The model under review builds one solid part; all positions refer to its coordinate system, in mm. A direction names the side the tool comes from. Round coordinates to 2 decimals unless told otherwise and drop trailing zeros. Loops run counter-clockwise (first coordinate to the right, second up) from the corner with the lowest first, then second, coordinate; pieces in that order, holes last. Notation, with made-up numbers: (-18.75, 88.5) - (-8.75, 88.5) arc R21 cw to (-8.75, 111.5) - close; hole circle Ø6 at (38, 30.5). An arc over 180 degrees is marked (long way). Answer as CSV lines item,"result".
from build123d import *

# Parameters (mm, degrees)
SKETCH2_R           = 6.465
BOSS_EXTRUDE1_DEPTH = 4.2
SKETCH3_R           = 7.74
BOSS_EXTRUDE2_DEPTH = 2.9
SKETCH4_R           = 6.0452
BOSS_EXTRUDE3_DEPTH = 10.25
SKETCH5_R           = 5.08
CUT_EXTRUDE1_DEPTH  = 15.45


with BuildPart() as part:
    # Sketch2 → Boss-Extrude1 (new body)
    with BuildSketch(Plane.XY):
        Circle(SKETCH2_R)
    extrude(amount=BOSS_EXTRUDE1_DEPTH)

    # Sketch3 → Boss-Extrude2 (add)
    with BuildSketch(Plane.XY.offset(4.2)):
        Circle(SKETCH3_R)
    extrude(amount=-BOSS_EXTRUDE2_DEPTH)

    # Sketch4 → Boss-Extrude3 (add)
    with BuildSketch(Plane.XY.offset(4.2)):
        Circle(SKETCH4_R)
    extrude(amount=BOSS_EXTRUDE3_DEPTH)

    # Sketch5 → Cut-Extrude1 (cut, through all)
    with BuildSketch(Plane.XY.offset(14.45)):
        Circle(SKETCH5_R)
    extrude(amount=-CUT_EXTRUDE1_DEPTH, mode=Mode.SUBTRACT)

    # Sketch6 → Cut-Revolve1 (revolve, cut)
    with BuildSketch(Plane(origin=(0, 0, 0), x_dir=(0, 0, -1), z_dir=(1, 0, 0))):
        Polygon((-14.45, 5.954405999), (-11.85, 6.0452), (-14.45, 6.0452), align=None)
    revolve(axis=Axis((0, 0, 0), (0, 0, 1)), mode=Mode.SUBTRACT)


solid = part.part
1. Take a section at C-C (z = 11). State the section outline as (x, y) points, plus the area to 3 significant figures.
Numbers:
outline,"circle Ø12.09 at (0, 0); hole circle Ø10.16 at (0, 0)"
area,"33.7 mm²"
2. Clearance check with flat-ended pins moving along their axes: pin 1 (3 mm diameter, centred on y = 6, z = 9, fed in from -X); pin 2 (1 mm diameter, centred on x = 5.5, z = 5.5, fed in from +Y); pin 3 (1 mm diameter, centred on x = -6, z = 3.5, fed in from -Y). State where each tip first meets the part, or that it passes through.
Numbers:
pin 1,"stops at x = -4.04"
pin 2,"stops at y = 3.4"
pin 3,"stops at y = -5.45"
3. Take a section at A-A (x = 0). State the section outline as (y, z) points (3 decimals), plus the area to 3 significant figures.
Numbers:
outline,"(-7.74, 1.3) - (-6.465, 1.3) - (-6.465, 0) - (-5.08, 0) - (-5.08, 14.45) - (-5.954, 14.45) - (-6.045, 11.85) - (-6.045, 4.2) - (-7.74, 4.2) - close; (5.08, 0) - (6.465, 0) - (6.465, 1.3) - (7.74, 1.3) - (7.74, 4.2) - (6.045, 4.2) - (6.045, 11.85) - (5.954, 14.45) - (5.08, 14.45) - close"
area,"38.6 mm²"
4. Tool access review of faces 1 (the face through (-5, -4, 4.2)), 2 (the face through (3.572, -6.867, 2.77)), 3 (the face through (-5, -5, 1.3)): name each direction out of +Z, -Z, +X, -X, +Y, -Y from which nothing blocks a thin tool from reaching the whole face with its end or side.
Numbers:
face 1,"+Z"
face 2,"+Z, -Z"
face 3,"-Z"
5. Take a section at D-D (z = 3.75). State the section outline as (x, y) points.
Numbers:
outline,"circle Ø15.48 at (0, 0); hole circle Ø10.16 at (0, 0)"
6. Wall thickness on probe 1 along Y at (x, z) = (0, 4); probe 2 along Y at (x, z) = (0, 9.5); probe 3 along Z at (x, y) = (2, -6.75): over which ranges is each line inside the solid? List them lowest first.
Numbers:
probe 1,"y = -7.74 to -5.08, 5.08 to 7.74"
probe 2,"y = -6.05 to -5.08, 5.08 to 6.05"
probe 3,"z = 1.3 to 4.2"
7. Draft analysis for pull direction Y (two halves, no side actions). For faces 4 (the face through (5, 2, 14.45)), 5 (the face through (5.766, 1.816, 7.971)), 6 (the face through (-0.661, 5.037, 7.326)), state which applies: +Y half, -Y half, draft (parallel to the pull), parting line (faces both ways), or undercut.
Numbers:
face 4,"draft"
face 5,"parting line"
face 6,"undercut"
